```python
from build123d import *

# Parameters (mm, degrees)
F0_R        = 15.875
F1_DEPTH    = 6.35
F2_W        = 9.525
F2_H        = 9.525
F3_DEPTH    = 62.23
F4_R        = 2.3876
F5_DEPTH    = 25.4
F6_T1_DEPTH = 62.23
F7_R        = 1.143


# Not quite as in the source:
# - a fillet or chamfer that OpenCascade refuses, or shapes differently, is made with other operations: its cross-section is extruded or revolved along the edge and cut away or added


with BuildPart() as f1:
    # F0 (on Right) → F1 (new body)
    with BuildSketch(Plane.YZ):
        Circle(F0_R)
    extrude(amount=F1_DEPTH)

    # F2 (on face) → F3 (join)
    with BuildSketch(Plane.YZ.offset(6.35)):
        with Locations((4.7625, 4.7625)):
            Rectangle(F2_W, F2_H)
        with Locations((-4.7625, -4.7625)):
            Rectangle(F2_W, F2_H)
        with Locations((-4.7625, 4.7625)):
            Rectangle(F2_W, F2_H)
        with Locations((4.7625, -4.7625)):
            Rectangle(F2_W, F2_H)
    extrude(amount=F3_DEPTH)

    # F4 (on face) → F5 (cut)
    with BuildSketch(Plane.XZ.offset(9.525)):
        with Locations((62.23, 0)):
            Circle(F4_R)
    extrude(amount=-F5_DEPTH, mode=Mode.SUBTRACT)

    # F6: fillet of radius 9.525 on 4 edges, made by hand

    # F6_s2 → F6_t1 (cut)
    with BuildSketch(Plane.YZ.offset(6.35)):
        with BuildLine():
            ThreePointArc((0, 9.525), (-6.7351920908, 6.7351920908), (-9.525, 0))
            Line((-9.525, 0), (-9.7155, 0))
            Line((-9.7155, 0), (-9.7155, 9.7155))
            Line((-9.7155, 9.7155), (0, 9.7155))
            Line((0, 9.7155), (0, 9.525))
        make_face()
        with BuildLine():
            ThreePointArc((0, 9.525), (6.7351920908, 6.7351920908), (9.525, 0))
            Line((9.525, 0), (9.7155, 0))
            Line((9.7155, 0), (9.7155, 9.7155))
            Line((9.7155, 9.7155), (0, 9.7155))
            Line((0, 9.7155), (0, 9.525))
        make_face()
        with BuildLine():
            ThreePointArc((-9.525, 0), (-6.7351920908, -6.7351920908), (0, -9.525))
            Line((0, -9.525), (0, -9.7155))
            Line((0, -9.7155), (-9.7155, -9.7155))
            Line((-9.7155, -9.7155), (-9.7155, 0))
            Line((-9.7155, 0), (-9.525, 0))
        make_face()
        with BuildLine():
            ThreePointArc((0, -9.525), (6.7351920908, -6.7351920908), (9.525, 0))
            Line((9.525, 0), (9.7155, 0))
            Line((9.7155, 0), (9.7155, -9.7155))
            Line((9.7155, -9.7155), (0, -9.7155))
            Line((0, -9.7155), (0, -9.525))
        make_face()
    extrude(amount=F6_T1_DEPTH, mode=Mode.SUBTRACT)

    # F7
    f7_edges = [f1.edges().sort_by_distance(p)[0] for p in [
        (68.58, -6.735192, -6.735192),
    ]]
    fillet(f7_edges, radius=F7_R)


solid = f1.part
```
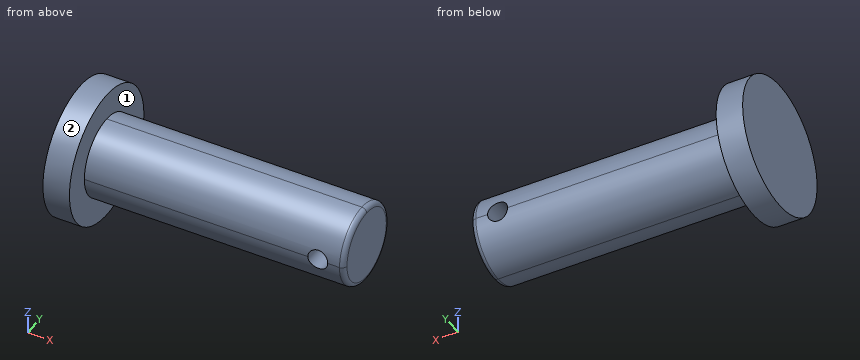
Input: part model. Units: mm. Frame: model coordinates. Face numbers are marked on the shaded views. A direction names the side the tool comes from. Give positions to 0.01 mm unless a question says otherwise; leave off trailing zeros. Order: outer loops, then holes, each group sorted by start corner. A loop starts at its lowest first (then second) coordinate and runs counter-clockwise, first axis right, second up.
1. Cut plane B-B (z = -11). Return loops of the section in (x, y), and give its area (3 significant figures).
Computed:
outline: (0, -11.45) - (6.35, -11.45) - (6.35, 11.45) - (0, 11.45) - close
area: 145 mm2
2. Pin query (flat end, axial travel): pin 1 Ø3 at (x, y) = (60.5, -5.5) entering from -Z; pin 2 Ø2 at (y, z) = (-9.5, -5.5) entering from +X; pin 3 Ø1 at (x, y) = (51, -10.5) entering from +Z; pin 4 Ø3 at (x, y) = (10, 1.5) entering from +Z (3 decimals). Return the tip coordinate at first contact, or that it passes through.
Computed:
pin 1: stops at z = -8.64
pin 2: stops at x = 6.35
pin 3: passes through
pin 4: stops at z = 9.525
3. Line query: probe 1 along X at (y, z) = (1.25, 0); probe 2 along Z at (x, y) = (62, 0) (1 decimal); probe 3 along X at (y, z) = (7.5, -8.5). Output: solid intervals per line, ascending.
Computed:
probe 1: x = 0 to 59.84, 64.62 to 68.58
probe 2: z = -9.5 to -2.4, 2.4 to 9.5
probe 3: x = 0 to 6.35
4. Cut plane C-C (y = -10.5). Return loops of the section in (x, z), and give its area (3 significant figures).
Computed:
outline: (0, -11.91) - (6.35, -11.91) - (6.35, 11.91) - (0, 11.91) - close
area: 151 mm2
5. Set-up query: the marked faces 1 and 2. Return all of +Z, -Z, +X, -X, +Y, -Y with unobstructed straight access to the full face (end or side cutting, diameter ignored); none if empty.
Computed:
face 1: +X
face 2: +X, -X
6. Cut plane A-A (x = 62.23). Return loops of the section in (y, z) (3 decimals), and give its area (3 significant figures).
Computed:
outline: (-9.221, -2.388) arc R9.525 ccw to (9.221, -2.388) - close; (-9.221, 2.388) - (9.221, 2.388) arc R9.525 ccw to start
area: 195 mm2
